Input: part model. Units: mm. Frame: model coordinates. A direction names the side the tool comes from. Round coordinates to 2 decimals unless told otherwise and drop trailing zeros. Loops run counter-clockwise (first coordinate to the right, second up) from the corner with the lowest first, then second, coordinate; pieces in that order, holes last. Notation, with made-up numbers: (22.5, 71.25) -> (37.5, 71.25) arc R23 cw to (37.5, 105.25) -> close; hole circle Ø9 at (16.5, 69). An arc over 180 degrees is marked (long way). Answer in a Markdown table with one row per item. Add a question column.
Q1. Section B-B, the plane x = 0. Output: boundary loops of the cut face in (y, z), and give its area (3 significant figures).
Q2. Section D-D, the plane z = -10. Output: boundary loops of the cut face in (x, y), and give its area (4 significant figures).
Q3. Pin query (flat end, axial travel): pin 1 (14 mm diameter, centred on x = -22.5, z = -35, fed in from +Y); pin 2 (4 mm diameter, centred on x = 28.5, y = -14, fed in from -Z); pin 3 (25 mm diameter, centred on x = 1, y = 3, fed in from -Z); pin 4 (12 mm diameter, centred on y = 9.5, z = -12.5, fed in from +X). Return the tip coordinate at first contact, or that it passes through.
Q4. Section C-C, the plane y = 0. Output: boundary loops of the cut face in (x, z), and give its area (3 significant figures).
Q5. Mould query, pull axis Z, two halves, no side actions, for faces 1 (the face through (0, 0, -18)), 2 (the face through (-37.5, -24, -25)), 3 (the face through (-2.75, -12.4, 9.37)), 4 (the face through (0, -5, 24.5)). Classes: pulls with the +Z half, pulls with the -Z half, needs draft (parallel to the pull), parting line crosses it, or undercut.
Q6. Ray query, L1, parallel to Z at x = 15, y = -6; L2, parallel to Z at x = -22.5, y = -20; L3, parallel to Y at x = -23.5, z = -13. Return the intervals inside material, ascending. Write a range as from..to.
Q7. Section A-A, the plane z = -34. Output: boundary loops of the cut face in (x, y), and give its area (3 significant figures).
Q8. Reachability of faces 5 (the face through (22.5, 0, -9)), 6 (the face through (-22.5, 0, -9)), 7 (the face through (23.846, 7.509, 21.712)), 8 (the face through (0, 17.5, -9)), 9 (the face through (-11.5, 5.9, 19)) from +Z, -Z, +X, -X, +Y, -Y: full face, straight path, thin tool, end or side. Return the list, or none.
```python
from build123d import *

# Parameters (mm, degrees)
F0_W      = 100
F0_H      = 35
F1_DEPTH  = 18
F2_R      = 12.7
F3_DEPTH  = 19
F4_R      = 25
F4_R_2    = 12.7
F5_DEPTH  = 5.5
F6_R      = 2.5
F7_DEPTH  = 3
F8_W      = 100
F8_H      = 57
F8_H_2    = 18
F9_DEPTH  = 12
F11_DEPTH = 50
F13_D     = 12
F13_DEPTH = 12
F14_W     = 15
F14_H     = 18
F15_DEPTH = 35


with BuildPart() as f1:
    # F0 (on Top) → F1 (new body)
    with BuildSketch(Plane.XY):
        Rectangle(F0_W, F0_H)
    extrude(amount=-F1_DEPTH)

    # F2 (on face) → F3 (join)
    with BuildSketch(Plane.XY):
        Circle(F2_R)
    extrude(amount=F3_DEPTH)

    # F4 (on face) → F5 (join)
    with BuildSketch(Plane.XY.offset(19)):
        Circle(F4_R)
        Circle(F4_R_2, mode=Mode.SUBTRACT)
        Circle(F4_R_2)
    extrude(amount=F5_DEPTH)

    # F6 (on face) → F7 (join)
    with BuildSketch(Plane.XY.offset(24.5)):
        Circle(F6_R)
    extrude(amount=F7_DEPTH)

    # F8 (on face) → F9 (join)
    with BuildSketch(Plane.XZ.offset(17.5)):
        with Locations((0, -46.5)):
            Rectangle(F8_W, F8_H)
        with Locations((0, -9)):
            Rectangle(F8_W, F8_H_2)
    extrude(amount=F9_DEPTH)

    # F10 (on face) → F11 (cut)
    with BuildSketch(Plane.XZ.offset(29.5)):
        Polygon((-37.5, -50), (-37.5, 0), (-50, 0), (-50, -75), (50, -75), (50, 0), (37.5, 0), (37.5, -50), align=None)
    extrude(amount=-F11_DEPTH, mode=Mode.SUBTRACT)

    # F13
    with Locations(Plane(origin=(0, -17.5, 0), x_dir=(-1, 0, 0), z_dir=(0, 1, 0))):
        with Locations((-22.5, -35), (22.5, -35)):
            Hole(F13_D / 2, depth=F13_DEPTH)

    # F14 (on face) → F15 (cut)
    with BuildSketch(Plane(origin=(0, 17.5, 0), x_dir=(-1, 0, 0), z_dir=(0, 1, 0))):
        with Locations((-30, -9)):
            Rectangle(F14_W, F14_H)
        with Locations((30, -9)):
            Rectangle(F14_W, F14_H)
    extrude(amount=-F15_DEPTH, mode=Mode.SUBTRACT)


solid = f1.part
```
Answer block:
| question | item | result |
|---|---|---|
| 1 | outline | (-29.5, -50) -> (-17.5, -50) -> (-17.5, -18) -> (17.5, -18) -> (17.5, 0) -> (12.7, 0) -> (12.7, 19) -> (25, 19) -> (25, 24.5) -> (2.5, 24.5) -> (2.5, 27.5) -> (-2.5, 27.5) -> (-2.5, 24.5) -> (-25, 24.5) -> (-25, 19) -> (-12.7, 19) -> (-12.7, 0) -> (-29.5, 0) -> close |
| 1 | area | 2,000 mm^2 |
| 2 | outline | (-37.5, -29.5) -> (37.5, -29.5) -> (37.5, -17.5) -> (22.5, -17.5) -> (22.5, 17.5) -> (-22.5, 17.5) -> (-22.5, -17.5) -> (-37.5, -17.5) -> close |
| 2 | area | 2,475 mm^2 |
| 3 | pin 1 | y = -17.5 |
| 3 | pin 2 | through |
| 3 | pin 3 | z = -18 |
| 3 | pin 4 | x = 22.5 |
| 4 | outline | (-25, 19) -> (-12.7, 19) -> (-12.7, 0) -> (-22.5, 0) -> (-22.5, -18) -> (22.5, -18) -> (22.5, 0) -> (12.7, 0) -> (12.7, 19) -> (25, 19) -> (25, 24.5) -> (2.5, 24.5) -> (2.5, 27.5) -> (-2.5, 27.5) -> (-2.5, 24.5) -> (-25, 24.5) -> close |
| 4 | area | 1,580 mm^2 |
| 5 | face 1 | pulls with the -Z half |
| 5 | face 2 | needs draft |
| 5 | face 3 | undercut |
| 5 | face 4 | pulls with the +Z half |
| 6 | L1 | -18..0, 19..24.5 |
| 6 | L2 | -50..-41, -29..0 |
| 6 | L3 | -29.5..-17.5 |
| 7 | outline | (-37.5, -29.5) -> (-28.42, -29.5) -> (-28.42, -17.5) -> (-37.5, -17.5) -> close; (-16.58, -29.5) -> (16.58, -29.5) -> (16.58, -17.5) -> (-16.58, -17.5) -> close; (28.42, -29.5) -> (37.5, -29.5) -> (37.5, -17.5) -> (28.42, -17.5) -> close |
| 7 | area | 616 mm^2 |
| 8 | face 5 | -Z, +X, +Y |
| 8 | face 6 | -Z, -X, +Y |
| 8 | face 7 | +Z |
| 8 | face 8 | -Z, +X, -X, +Y |
| 8 | face 9 | none |
